Part model, mm, in its own coordinate system. Give positions to 0.01 mm unless a question says otherwise; leave off trailing zeros. Order: outer loops, then holes, each group sorted by start corner. A loop starts at its lowest first (then second) coordinate and runs counter-clockwise, first axis right, second up. Notation, with made-up numbers: M -32,65.5 L 3,65.5 A26 cw 3,84.5 Z; hole C 66,64 d2. An arc over 180 degrees is marked long. Answer as a JSON object with one key per item and string values.
from build123d import *

# Parameters (mm, degrees)
SKETCH1_W           = 50.8
SKETCH1_H           = 25.4
SKETCH1_W_2         = 44.45
SKETCH1_H_2         = 19.05
BOSS_EXTRUDE1_DEPTH = 279.4
CUT_EXTRUDE1_REACH  = 283.7
SKETCH2_R           = 2.54


with BuildPart() as part:
    # Sketch1 → Boss-Extrude1 (new body)
    with BuildSketch(Plane.XY):
        Rectangle(SKETCH1_W, SKETCH1_H)
        Rectangle(SKETCH1_W_2, SKETCH1_H_2, mode=Mode.SUBTRACT)
    extrude(amount=BOSS_EXTRUDE1_DEPTH)

    # Cut-Extrude1: up to this face of the body (flat: up to its plane)
    cut_extrude1_end = Plane(part.part.faces().sort_by_distance((0, -12.7, 139.7))[0])
    # Sketch2 → Cut-Extrude1 (cut, up to the picked face)
    with BuildSketch(Plane(origin=(0, 12.7, 0), x_dir=(1, 0, 0), z_dir=(0, 1, 0)), mode=Mode.PRIVATE) as cut_extrude1_sk1:
        with Locations(Location((-12.7, -3.81, 0), (0, 0, 270))):
            Circle(SKETCH2_R)
    cut_extrude1_tool1 = split(extrude(cut_extrude1_sk1.sketch, amount=-CUT_EXTRUDE1_REACH, mode=Mode.PRIVATE), bisect_by=cut_extrude1_end, keep=Keep.BOTH, mode=Mode.PRIVATE)
    # Sketch2 → Cut-Extrude1 (cut, up to the picked face)
    with BuildSketch(Plane(origin=(0, 12.7, 0), x_dir=(1, 0, 0), z_dir=(0, 1, 0)), mode=Mode.PRIVATE) as cut_extrude1_sk2:
        with Locations(Location((-12.7, -266.7, 0), (0, 0, 270))):
            Circle(SKETCH2_R)
    cut_extrude1_tool2 = split(extrude(cut_extrude1_sk2.sketch, amount=-CUT_EXTRUDE1_REACH, mode=Mode.PRIVATE), bisect_by=cut_extrude1_end, keep=Keep.BOTH, mode=Mode.PRIVATE)
    # Sketch2 → Cut-Extrude1 (cut, up to the picked face)
    with BuildSketch(Plane(origin=(0, 12.7, 0), x_dir=(1, 0, 0), z_dir=(0, 1, 0)), mode=Mode.PRIVATE) as cut_extrude1_sk3:
        with Locations(Location((12.7, -266.7, 0), (0, 0, 270))):
            Circle(SKETCH2_R)
    cut_extrude1_tool3 = split(extrude(cut_extrude1_sk3.sketch, amount=-CUT_EXTRUDE1_REACH, mode=Mode.PRIVATE), bisect_by=cut_extrude1_end, keep=Keep.BOTH, mode=Mode.PRIVATE)
    # Sketch2 → Cut-Extrude1 (cut, up to the picked face)
    with BuildSketch(Plane(origin=(0, 12.7, 0), x_dir=(1, 0, 0), z_dir=(0, 1, 0)), mode=Mode.PRIVATE) as cut_extrude1_sk4:
        with Locations(Location((12.7, -241.3, 0), (0, 0, 270))):
            Circle(SKETCH2_R)
    cut_extrude1_tool4 = split(extrude(cut_extrude1_sk4.sketch, amount=-CUT_EXTRUDE1_REACH, mode=Mode.PRIVATE), bisect_by=cut_extrude1_end, keep=Keep.BOTH, mode=Mode.PRIVATE)
    # Sketch2 → Cut-Extrude1 (cut, up to the picked face)
    with BuildSketch(Plane(origin=(0, 12.7, 0), x_dir=(1, 0, 0), z_dir=(0, 1, 0)), mode=Mode.PRIVATE) as cut_extrude1_sk5:
        with Locations(Location((12.7, -215.9, 0), (0, 0, 270))):
            Circle(SKETCH2_R)
    cut_extrude1_tool5 = split(extrude(cut_extrude1_sk5.sketch, amount=-CUT_EXTRUDE1_REACH, mode=Mode.PRIVATE), bisect_by=cut_extrude1_end, keep=Keep.BOTH, mode=Mode.PRIVATE)
    # Sketch2 → Cut-Extrude1 (cut, up to the picked face)
    with BuildSketch(Plane(origin=(0, 12.7, 0), x_dir=(1, 0, 0), z_dir=(0, 1, 0)), mode=Mode.PRIVATE) as cut_extrude1_sk6:
        with Locations(Location((12.7, -190.5, 0), (0, 0, 270))):
            Circle(SKETCH2_R)
    cut_extrude1_tool6 = split(extrude(cut_extrude1_sk6.sketch, amount=-CUT_EXTRUDE1_REACH, mode=Mode.PRIVATE), bisect_by=cut_extrude1_end, keep=Keep.BOTH, mode=Mode.PRIVATE)
    # Sketch2 → Cut-Extrude1 (cut, up to the picked face)
    with BuildSketch(Plane(origin=(0, 12.7, 0), x_dir=(1, 0, 0), z_dir=(0, 1, 0)), mode=Mode.PRIVATE) as cut_extrude1_sk7:
        with Locations(Location((12.7, -165.1, 0), (0, 0, 270))):
            Circle(SKETCH2_R)
    cut_extrude1_tool7 = split(extrude(cut_extrude1_sk7.sketch, amount=-CUT_EXTRUDE1_REACH, mode=Mode.PRIVATE), bisect_by=cut_extrude1_end, keep=Keep.BOTH, mode=Mode.PRIVATE)
    # Sketch2 → Cut-Extrude1 (cut, up to the picked face)
    with BuildSketch(Plane(origin=(0, 12.7, 0), x_dir=(1, 0, 0), z_dir=(0, 1, 0)), mode=Mode.PRIVATE) as cut_extrude1_sk8:
        with Locations(Location((-12.7, -241.3, 0), (0, 0, 270))):
            Circle(SKETCH2_R)
    cut_extrude1_tool8 = split(extrude(cut_extrude1_sk8.sketch, amount=-CUT_EXTRUDE1_REACH, mode=Mode.PRIVATE), bisect_by=cut_extrude1_end, keep=Keep.BOTH, mode=Mode.PRIVATE)
    # Sketch2 → Cut-Extrude1 (cut, up to the picked face)
    with BuildSketch(Plane(origin=(0, 12.7, 0), x_dir=(1, 0, 0), z_dir=(0, 1, 0)), mode=Mode.PRIVATE) as cut_extrude1_sk9:
        with Locations(Location((-12.7, -215.9, 0), (0, 0, 270))):
            Circle(SKETCH2_R)
    cut_extrude1_tool9 = split(extrude(cut_extrude1_sk9.sketch, amount=-CUT_EXTRUDE1_REACH, mode=Mode.PRIVATE), bisect_by=cut_extrude1_end, keep=Keep.BOTH, mode=Mode.PRIVATE)
    # Sketch2 → Cut-Extrude1 (cut, up to the picked face)
    with BuildSketch(Plane(origin=(0, 12.7, 0), x_dir=(1, 0, 0), z_dir=(0, 1, 0)), mode=Mode.PRIVATE) as cut_extrude1_sk10:
        with Locations(Location((-12.7, -190.5, 0), (0, 0, 270))):
            Circle(SKETCH2_R)
    cut_extrude1_tool10 = split(extrude(cut_extrude1_sk10.sketch, amount=-CUT_EXTRUDE1_REACH, mode=Mode.PRIVATE), bisect_by=cut_extrude1_end, keep=Keep.BOTH, mode=Mode.PRIVATE)
    # Sketch2 → Cut-Extrude1 (cut, up to the picked face)
    with BuildSketch(Plane(origin=(0, 12.7, 0), x_dir=(1, 0, 0), z_dir=(0, 1, 0)), mode=Mode.PRIVATE) as cut_extrude1_sk11:
        with Locations(Location((-12.7, -165.1, 0), (0, 0, 270))):
            Circle(SKETCH2_R)
    cut_extrude1_tool11 = split(extrude(cut_extrude1_sk11.sketch, amount=-CUT_EXTRUDE1_REACH, mode=Mode.PRIVATE), bisect_by=cut_extrude1_end, keep=Keep.BOTH, mode=Mode.PRIVATE)
    # Sketch2 → Cut-Extrude1 (cut, up to the picked face)
    with BuildSketch(Plane(origin=(0, 12.7, 0), x_dir=(1, 0, 0), z_dir=(0, 1, 0)), mode=Mode.PRIVATE) as cut_extrude1_sk12:
        with Locations(Location((12.7, -3.81, 0), (0, 0, 270))):
            Circle(SKETCH2_R)
    cut_extrude1_tool12 = split(extrude(cut_extrude1_sk12.sketch, amount=-CUT_EXTRUDE1_REACH, mode=Mode.PRIVATE), bisect_by=cut_extrude1_end, keep=Keep.BOTH, mode=Mode.PRIVATE)
    # Sketch2 → Cut-Extrude1 (cut, up to the picked face)
    with BuildSketch(Plane(origin=(0, 12.7, 0), x_dir=(1, 0, 0), z_dir=(0, 1, 0)), mode=Mode.PRIVATE) as cut_extrude1_sk13:
        with Locations(Location((12.7, -29.21, 0), (0, 0, 270))):
            Circle(SKETCH2_R)
    cut_extrude1_tool13 = split(extrude(cut_extrude1_sk13.sketch, amount=-CUT_EXTRUDE1_REACH, mode=Mode.PRIVATE), bisect_by=cut_extrude1_end, keep=Keep.BOTH, mode=Mode.PRIVATE)
    # Sketch2 → Cut-Extrude1 (cut, up to the picked face)
    with BuildSketch(Plane(origin=(0, 12.7, 0), x_dir=(1, 0, 0), z_dir=(0, 1, 0)), mode=Mode.PRIVATE) as cut_extrude1_sk14:
        with Locations(Location((12.7, -54.61, 0), (0, 0, 270))):
            Circle(SKETCH2_R)
    cut_extrude1_tool14 = split(extrude(cut_extrude1_sk14.sketch, amount=-CUT_EXTRUDE1_REACH, mode=Mode.PRIVATE), bisect_by=cut_extrude1_end, keep=Keep.BOTH, mode=Mode.PRIVATE)
    # Sketch2 → Cut-Extrude1 (cut, up to the picked face)
    with BuildSketch(Plane(origin=(0, 12.7, 0), x_dir=(1, 0, 0), z_dir=(0, 1, 0)), mode=Mode.PRIVATE) as cut_extrude1_sk15:
        with Locations(Location((-12.7, -29.21, 0), (0, 0, 270))):
            Circle(SKETCH2_R)
    cut_extrude1_tool15 = split(extrude(cut_extrude1_sk15.sketch, amount=-CUT_EXTRUDE1_REACH, mode=Mode.PRIVATE), bisect_by=cut_extrude1_end, keep=Keep.BOTH, mode=Mode.PRIVATE)
    # Sketch2 → Cut-Extrude1 (cut, up to the picked face)
    with BuildSketch(Plane(origin=(0, 12.7, 0), x_dir=(1, 0, 0), z_dir=(0, 1, 0)), mode=Mode.PRIVATE) as cut_extrude1_sk16:
        with Locations(Location((-12.7, -54.61, 0), (0, 0, 270))):
            Circle(SKETCH2_R)
    cut_extrude1_tool16 = split(extrude(cut_extrude1_sk16.sketch, amount=-CUT_EXTRUDE1_REACH, mode=Mode.PRIVATE), bisect_by=cut_extrude1_end, keep=Keep.BOTH, mode=Mode.PRIVATE)
    # Sketch2 → Cut-Extrude1 (cut, up to the picked face)
    with BuildSketch(Plane(origin=(0, 12.7, 0), x_dir=(1, 0, 0), z_dir=(0, 1, 0)), mode=Mode.PRIVATE) as cut_extrude1_sk17:
        with Locations(Location((-12.7, -80.01, 0), (0, 0, 270))):
            Circle(SKETCH2_R)
    cut_extrude1_tool17 = split(extrude(cut_extrude1_sk17.sketch, amount=-CUT_EXTRUDE1_REACH, mode=Mode.PRIVATE), bisect_by=cut_extrude1_end, keep=Keep.BOTH, mode=Mode.PRIVATE)
    # Sketch2 → Cut-Extrude1 (cut, up to the picked face)
    with BuildSketch(Plane(origin=(0, 12.7, 0), x_dir=(1, 0, 0), z_dir=(0, 1, 0)), mode=Mode.PRIVATE) as cut_extrude1_sk18:
        with Locations(Location((12.7, -80.01, 0), (0, 0, 270))):
            Circle(SKETCH2_R)
    cut_extrude1_tool18 = split(extrude(cut_extrude1_sk18.sketch, amount=-CUT_EXTRUDE1_REACH, mode=Mode.PRIVATE), bisect_by=cut_extrude1_end, keep=Keep.BOTH, mode=Mode.PRIVATE)
    add(cut_extrude1_tool1.solids().sort_by(Axis((-12.7, 12.7, 3.81), (0, -1, 0)))[0], mode=Mode.SUBTRACT)
    add(cut_extrude1_tool2.solids().sort_by(Axis((-12.7, 12.7, 266.7), (0, -1, 0)))[0], mode=Mode.SUBTRACT)
    add(cut_extrude1_tool3.solids().sort_by(Axis((12.7, 12.7, 266.7), (0, -1, 0)))[0], mode=Mode.SUBTRACT)
    add(cut_extrude1_tool4.solids().sort_by(Axis((12.7, 12.7, 241.3), (0, -1, 0)))[0], mode=Mode.SUBTRACT)
    add(cut_extrude1_tool5.solids().sort_by(Axis((12.7, 12.7, 215.9), (0, -1, 0)))[0], mode=Mode.SUBTRACT)
    add(cut_extrude1_tool6.solids().sort_by(Axis((12.7, 12.7, 190.5), (0, -1, 0)))[0], mode=Mode.SUBTRACT)
    add(cut_extrude1_tool7.solids().sort_by(Axis((12.7, 12.7, 165.1), (0, -1, 0)))[0], mode=Mode.SUBTRACT)
    add(cut_extrude1_tool8.solids().sort_by(Axis((-12.7, 12.7, 241.3), (0, -1, 0)))[0], mode=Mode.SUBTRACT)
    add(cut_extrude1_tool9.solids().sort_by(Axis((-12.7, 12.7, 215.9), (0, -1, 0)))[0], mode=Mode.SUBTRACT)
    add(cut_extrude1_tool10.solids().sort_by(Axis((-12.7, 12.7, 190.5), (0, -1, 0)))[0], mode=Mode.SUBTRACT)
    add(cut_extrude1_tool11.solids().sort_by(Axis((-12.7, 12.7, 165.1), (0, -1, 0)))[0], mode=Mode.SUBTRACT)
    add(cut_extrude1_tool12.solids().sort_by(Axis((12.7, 12.7, 3.81), (0, -1, 0)))[0], mode=Mode.SUBTRACT)
    add(cut_extrude1_tool13.solids().sort_by(Axis((12.7, 12.7, 29.21), (0, -1, 0)))[0], mode=Mode.SUBTRACT)
    add(cut_extrude1_tool14.solids().sort_by(Axis((12.7, 12.7, 54.61), (0, -1, 0)))[0], mode=Mode.SUBTRACT)
    add(cut_extrude1_tool15.solids().sort_by(Axis((-12.7, 12.7, 29.21), (0, -1, 0)))[0], mode=Mode.SUBTRACT)
    add(cut_extrude1_tool16.solids().sort_by(Axis((-12.7, 12.7, 54.61), (0, -1, 0)))[0], mode=Mode.SUBTRACT)
    add(cut_extrude1_tool17.solids().sort_by(Axis((-12.7, 12.7, 80.01), (0, -1, 0)))[0], mode=Mode.SUBTRACT)
    add(cut_extrude1_tool18.solids().sort_by(Axis((12.7, 12.7, 80.01), (0, -1, 0)))[0], mode=Mode.SUBTRACT)


solid = part.part
1. Cut at B-B on z = 29.21. Give the cut face in (x, y) (3 decimals), plus the area to 3 significant figures.
Worked answers:
{"outline": "M -25.4,-12.7 L -15.24,-12.7 L -15.24,-9.525 L -22.225,-9.525 L -22.225,9.525 L -15.24,9.525 L -15.24,12.7 L -25.4,12.7 Z; M -10.16,-12.7 L 10.16,-12.7 L 10.16,-9.525 L -10.16,-9.525 Z; M -10.16,9.525 L 10.16,9.525 L 10.16,12.7 L -10.16,12.7 Z; M 15.24,-12.7 L 25.4,-12.7 L 25.4,12.7 L 15.24,12.7 L 15.24,9.525 L 22.225,9.525 L 22.225,-9.525 L 15.24,-9.525 Z", "area": "379 mm^2"}
2. Cut at A-A on x = 1.5. Give the cut face in (y, z) (3 decimals).
Worked answers:
{"outline": "M -12.7,0 L -9.525,0 L -9.525,279.4 L -12.7,279.4 Z; M 9.525,0 L 12.7,0 L 12.7,279.4 L 9.525,279.4 Z"}
3. Two-plate mould, pull along X, no slides. Class faces 1 (the flat face through (0, 10, 279.4)), 2 (the cylindrical face through (15.22, -11.09, 3.48)), 3 (the cylindrical face through (-11.937, -11.09, 167.523)): +X half, -X half, draft (parallel to the pull), parting line (faces both ways), or undercut.
Worked answers:
{"face 1": "draft", "face 2": "undercut", "face 3": "undercut"}
4. Cut at C-C on y = -6. Give the cut face in (x, z) (3 decimals).
Worked answers:
{"outline": "M -25.4,0 L -22.225,0 L -22.225,279.4 L -25.4,279.4 Z; M 22.225,0 L 25.4,0 L 25.4,279.4 L 22.225,279.4 Z"}
5. Probe line 1 along X through (y, z) = (-11.85, 80.01); line 2 along Y through (x, z) = (21.5, 208.5) (3 decimals); line 3 along X through (y, z) = (-3, 124.5) (3 decimals). List the from-to ranges inside material, lowest first.
Worked answers:
{"line 1": "x = -25.4 to -15.24, -10.16 to 10.16, 15.24 to 25.4", "line 2": "y = -12.7 to -9.525, 9.525 to 12.7", "line 3": "x = -25.4 to -22.225, 22.225 to 25.4"}
6. Cut at D-D on x = 12.7. State how many separate pieces and enclosed holes the cut face has, plus the area to 3 significant figures.
Worked answers:
{"separate pieces": "20", "enclosed holes": "0", "area": "1,480 mm^2"}
